```python
from build123d import *

# Parameters (mm, degrees)
SKETCH1_R           = 75
BOSS_EXTRUDE1_DEPTH = 6
SKETCH2_R           = 32.5
CUT_EXTRUDE1_DEPTH  = 107.235587258
SKETCH3_R           = 3.390748994
CUT_EXTRUDE2_DEPTH  = 5.204728
CIRPATTERN1_START   = 0.79527246
CIRPATTERN1_DEPTH   = 5.20472754


# Read off the part's stored shape, not the designer's step: CirPattern1
with BuildPart() as part:
    # Sketch1 → Boss-Extrude1 (new body)
    with BuildSketch(Plane(origin=(0, 0, 0), x_dir=(1, 0, 0), z_dir=(0, 1, 0))):
        with Locations(Location((0, 0, 0), (0, 0, 270))):
            Circle(SKETCH1_R)
    extrude(amount=BOSS_EXTRUDE1_DEPTH)

    # Sketch2 → Cut-Extrude1 (cut, through all)
    with BuildSketch(Plane(origin=(0, 0, 0), x_dir=(1, 0, 0), z_dir=(0, 1, 0))):
        with Locations(Location((0, 0, 0), (0, 0, 270))):
            Circle(SKETCH2_R)
    extrude(amount=CUT_EXTRUDE1_DEPTH, mode=Mode.SUBTRACT)

    # Sketch3 → Cut-Extrude2 (cut)
    with BuildSketch(Plane(origin=(0, 6, 0), x_dir=(1, 0, 0), z_dir=(0, 1, 0))):
        with Locations((-31.034865261, 0)):
            Circle(SKETCH3_R)
    extrude(amount=-CUT_EXTRUDE2_DEPTH, mode=Mode.SUBTRACT)

    # CirPattern1 outline → CirPattern1 (cut)
    with BuildSketch(Plane(origin=(0, 0, 0), x_dir=(1, 0, 0), z_dir=(0, 1, 0)).offset(CIRPATTERN1_START)):
        with BuildLine():
            ThreePointArc((-13.46783867, -29.578156156), (-16.25, -28.145825623), (-18.881515293, -26.4525685))
            ThreePointArc((-18.881515293, -26.4525685), (-17.212807128, -29.813456486), (-13.46783867, -29.578156156))
        make_face()
        with BuildLine():
            ThreePointArc((-13.46783867, 29.578156156), (-17.212807128, 29.813456486), (-18.881515293, 26.4525685))
            ThreePointArc((-18.881515293, 26.4525685), (-16.25, 28.145825623), (-13.46783867, 29.578156156))
        make_face()
        with BuildLine():
            ThreePointArc((18.881515293, -26.4525685), (16.25, -28.145825623), (13.46783867, -29.578156156))
            ThreePointArc((13.46783867, -29.578156156), (17.212807128, -29.813456486), (18.881515293, -26.4525685))
        make_face()
        with BuildLine():
            ThreePointArc((18.881515293, 26.4525685), (17.212807128, 29.813456486), (13.46783867, 29.578156156))
            ThreePointArc((13.46783867, 29.578156156), (16.25, 28.145825623), (18.881515293, 26.4525685))
        make_face()
        with BuildLine():
            ThreePointArc((32.349353963, 3.125587656), (32.5, 0), (32.349353963, -3.125587656))
            ThreePointArc((32.349353963, -3.125587656), (34.425614255, 0), (32.349353963, 3.125587656))
        make_face()
    extrude(amount=CIRPATTERN1_DEPTH, mode=Mode.SUBTRACT)


solid = part.part
```
The model under review builds one solid part; all positions refer to its coordinate system, in mm. A direction names the side the tool comes from. Coordinates: 2 decimals unless noted, no trailing zeros. Write each loop counter-clockwise with the first axis right and the second up, starting at its lowest first coordinate (ties: lowest second). Pieces come first, ordered by that corner, then holes. Notation, with made-up numbers: (16, 8) - (55, 8) arc R11 ccw to (55, 12) - close; hole circle Ø9 at (81, 56). An arc over 180 degrees is marked (long way). Write item = value, one per line.
(1) Consider section C-C, the plane y = 2.2. Give the boundary of the cut face in (x, z).
Result sheet:
outline = circle Ø150 at (0, 0); hole (-32.35, -3.13) arc R32.5 ccw to (-18.88, -26.45) arc R3.39 ccw to (-13.47, -29.58) arc R32.5 ccw to (13.47, -29.58) arc R3.39 ccw to (18.88, -26.45) arc R32.5 ccw to (32.35, -3.13) arc R3.39 ccw to (32.35, 3.13) arc R32.5 ccw to (18.88, 26.45) arc R3.39 ccw to (13.47, 29.58) arc R32.5 ccw to (-13.47, 29.58) arc R3.39 ccw to (-18.88, 26.45) arc R32.5 ccw to (-32.35, 3.13) arc R3.39 ccw to start
(2) Mouldability with a two-part tool opening along X and no side actions: class faces 1 (the face through (-45.636, 2.958, -59.517)), 2 (the face through (9.76, 2.96, 31)), 3 (the face through (-32, 0, 16)) as pulls with the +X half, pulls with the -X half, needs draft (parallel to the pull), parting line crosses it, or undercut.
Result sheet:
face_1 = parting line crosses it
face_2 = undercut
face_3 = needs draft
(3) Consider section D-D, the plane x = 17. Give the boundary of the cut face in (y, z), then the cut area to 3 significant figures.
Result sheet:
outline = (0, -73.05) - (6, -73.05) - (6, -29.93) - (0.8, -29.93) - (0.8, -27.7) - (0, -27.7) - close; (0, 27.7) - (0.8, 27.7) - (0.8, 29.93) - (6, 29.93) - (6, 73.05) - (0, 73.05) - close
area = 521 mm^2
(4) Consider section B-B, the plane x = 0. Give the boundary of the cut face in (y, z), then the cut area to 3 significant figures.
Result sheet:
outline = (0, -75) - (6, -75) - (6, -32.5) - (0, -32.5) - close; (0, 32.5) - (6, 32.5) - (6, 75) - (0, 75) - close
area = 510 mm^2
(5) For line 1 (X direction, y = 2.15, z = 0); line 2 (Z direction, x = 1.5, y = 2.6) (3 decimals); line 3 (Z direction, x = -9, y = 4.1), list the stretches that pass through material, from the lowest coordinate up. Write a range as [from, to].
Result sheet:
line_1 = [-75, -34.43], [34.43, 75]
line_2 = [-74.985, -32.465], [32.465, 74.985]
line_3 = [-74.46, -31.23], [31.23, 74.46]
(6) For P1, Ø1.1, axis at x = 16, z = -28, coming from the +Y side; P2, Ø3, axis at y = 4, z = -48, coming from the +X side, all flat-tipped, find the tip position at first contact; note any pin that passes through.
Result sheet:
P1 = 0.8
P2 = 58.85
(7) Consider section A-A, the plane z = 0. Give the boundary of the cut face in (x, y).
Result sheet:
outline = (-75, 0) - (-32.5, 0) - (-32.5, 0.8) - (-34.43, 0.8) - (-34.43, 6) - (-75, 6) - close; (32.5, 0) - (75, 0) - (75, 6) - (34.43, 6) - (34.43, 0.8) - (32.5, 0.8) - close
(8) Machinability: for faces 4 (the face through (-32, 6, 16)), 5 (the face through (-17.261, 3.361, 29.785)), which of the approach directions +Z, -Z, +X, -X, +Y, -Y give a long, thin tool a straight path to every point of the face, cutting with its end or side? Answer none if there is none.
Result sheet:
face_4 = +Z, -Z, +X, -X, +Y
face_5 = +Y
